Check sheet for the modelled part. Datum: model origin and axes. Units: mm. A direction names the side the tool comes from. Give positions to 0.01 mm unless a question says otherwise; leave off trailing zeros. Loops run counter-clockwise (first coordinate to the right, second up) from the corner with the lowest first, then second, coordinate; pieces in that order, holes last. Notation, with made-up numbers: (-27.5, 15.25) -> (-16.5, 15.25) arc R10 cw to (-16.5, 20.25) -> close; hole circle Ø4 at (54.5, 4). An arc over 180 degrees is marked (long way). Write each question's results on one line, items separated by ' | '. Start each with the question number.
Item 1: Mould release check, pull along X, two halves, no side actions. Record for faces 3 (the face through (11.92, 37.546, -7.195)), 4 (the face through (0, 0, 0)), 5 (the face through (17.48, 19.77, 3.88)): pulls with the +X half, pulls with the -X half, needs draft (parallel to the pull), parting line crosses it, or undercut.
Item 2: Gauge pin test, flat ends, axial feed: pin 1 Ø6 at (x, z) = (6.5, 12) entering from +Y; pin 2 Ø1.5 at (x, z) = (11, 6.35) entering from -Y; pin 3 Ø1 at (y, z) = (28, 13.5) entering from +X; pin 4 Ø2 at (x, z) = (11, -6.35) entering from +Y. Record the tip position at first contact, or that the pin passes through.
Item 3: Access from +Z, -Z, +X, -X, +Y, -Y to the whole of each face (thin tool, end or side, straight path). Record for faces 1 (the face through (0.27, 37.55, 13.92)), 2 (the face through (0, 55.423, 0)).
Item 4: Scan lines: line 1 along Y through (x, z) = (14, 2); line 2 along X through (y, z) = (38.2, -12.7); line 3 along X through (y, z) = (39.15, 12.7). Record each from-to range of solid material in increasing order.
Item 5: Cross-section at C-C on y = 21.5. Enter the section's corners in (x, z), then the cut area to 3 significant figures.
Item 6: Cross-section at B-B on y = 44.5. Enter the section's corners in (x, z), then the cut area to 3 significant figures.
Item 7: Cross-section at A-A on z = 0. Enter the section's corners in (x, y).
from build123d import *

# Parameters (mm, degrees)
SKETCH1_R                           = 17.907
BOSS_EXTRUDE1_DEPTH                 = 40.0812
M3X0_5_BOTTOMING_TAPPED_HOLE1_D     = 2.5
M3X0_5_BOTTOMING_TAPPED_HOLE1_DEPTH = 5
M3X0_5_BOTTOMING_TAPPED_HOLE1_TIP   = 0.751075774
SKETCH4_R                           = 1.58
BOSS_EXTRUDE2_DEPTH                 = 15.3416
CHAMFER1_SIZE                       = 1


with BuildPart() as part:
    # Sketch1 → Boss-Extrude1 (new body)
    with BuildSketch(Plane(origin=(0, 0, 0), x_dir=(1, 0, 0), z_dir=(0, 1, 0))):
        with Locations(Location((0, 0, 0), (0, 0, 90))):
            Circle(SKETCH1_R)
    extrude(amount=BOSS_EXTRUDE1_DEPTH)

    # M3x0.5 Bottoming Tapped Hole1
    with Locations(Plane(origin=(0, 40.0812, 0), x_dir=(1, 0, 0), z_dir=(0, 1, 0))):
        with Locations((0, 12.7), (10.998522628, 6.35), (10.998522628, -6.35), (0, -12.7), (-10.998522628, -6.35), (-10.998522628, 6.35)):
            Hole(M3X0_5_BOTTOMING_TAPPED_HOLE1_D / 2, depth=M3X0_5_BOTTOMING_TAPPED_HOLE1_DEPTH)
            with Locations((0, 0, -(M3X0_5_BOTTOMING_TAPPED_HOLE1_DEPTH + M3X0_5_BOTTOMING_TAPPED_HOLE1_TIP / 2))):  # 118° drill point
                Cone(0, M3X0_5_BOTTOMING_TAPPED_HOLE1_D / 2, M3X0_5_BOTTOMING_TAPPED_HOLE1_TIP, mode=Mode.SUBTRACT)

    # Sketch4 → Boss-Extrude2 (add)
    with BuildSketch(Plane(origin=(0, 40.0812, 0), x_dir=(1, 0, 0), z_dir=(0, 1, 0))):
        with Locations(Location((0, 0, 0), (0, 0, 270))):
            Circle(SKETCH4_R)
    extrude(amount=BOSS_EXTRUDE2_DEPTH)

    # Chamfer1
    chamfer1_edges = [part.edges().sort_by_distance(p)[0] for p in [
        (0, 0, 17.907),
        (0, 40.0812, 17.907),
    ]]
    chamfer(chamfer1_edges, length=CHAMFER1_SIZE)


solid = part.part
Answer sheet:
1) face 3: undercut | face 4: needs draft | face 5: parting line crosses it
2) pin 1: stops at y = 40.08 | pin 2: stops at y = 0 | pin 3: stops at x = 12.32 | pin 4: stops at y = 34.93
3) face 1: +Y | face 2: +Z, -Z, +X, -X, +Y
4) line 1: y = 0 to 40.08 | line 2: x = -12.62 to -1.25, 1.25 to 12.62 | line 3: x = -12.53 to -1.25, 1.25 to 12.53
5) outline: circle Ø35.81 at (0, 0) | area: 1,010 mm²
6) outline: circle Ø3.16 at (0, 0) | area: 7.84 mm²
7) outline: (-17.91, 1) -> (-16.91, 0) -> (16.91, 0) -> (17.91, 1) -> (17.91, 39.08) -> (16.91, 40.08) -> (1.58, 40.08) -> (1.58, 55.42) -> (-1.58, 55.42) -> (-1.58, 40.08) -> (-16.91, 40.08) -> (-17.91, 39.08) -> close
